Check sheet for the modelled part. Datum: model origin and axes. Units: mm. A direction names the side the tool comes from. Round coordinates to 2 decimals unless told otherwise and drop trailing zeros. Order: outer loops, then holes, each group sorted by start corner. A loop starts at its lowest first (then second) coordinate and runs counter-clockwise, first axis right, second up.
Q1. Cross-section at A-A on y = 0. Record the cut outline in (x, z).
Q2. Set-up check for faces 1 (the flat face through (0, 3, 19)), 2 (the cylindrical face through (-6, 0, 21)), 3 (the flat face through (0, -6, 14)): record each of +Z, -Z, +X, -X, +Y, -Y from which the full face is reachable in a straight line by a thin tool's end or side.
Q3. Scan lines: probe 1 along Y at (x, z) = (13.5, 18.5); probe 2 along Y at (x, z) = (-5, 16); probe 3 along X at (y, z) = (4, 18.75). Record each from-to range of solid material in increasing order.
Q4. Depth check by flat-ended pin: P1, Ø4, axis at x = 0, z = 17.5, coming from the -Y side; P2, Ø2, axis at x = -18, z = 17.5, coming from the +Y side; P3, Ø23, axis at x = -10.58, y = -14.56, coming from the +Z side. Enter the tip coordinate at first touch or a pass-through.
Q5. Cross-section at B-B on x = -13. Give the number of separate pieces and of enclosed holes in the cut face, then the cut area to 3 significant figures.
Q6. Mould release check, pull along Y, two halves, no side actions. Record for faces 4 (the flat face through (-1.42, -3.92, 24)), 5 (the cylindrical face through (-1.302, 27.915, 16.465)), 6 (the cylindrical face through (22.923, -2.581, 16.465)), 7 (the cylindrical face through (-29.97, 1.32, 16.5)): +Y half, -Y half, draft (parallel to the pull), parting line (faces both ways), or undercut.
from build123d import *

# Parameters (mm, degrees)
CYLINDER003_R     = 10
CYLINDER003_DEPTH = 10
ARRAY_COUNT       = 5
TORUS001_R        = 0.8
TORUS_R           = 0.8
CYLINDER_R        = 4
CYLINDER_DEPTH    = 10
BOX_W             = 8
BOX_H             = 7
BOX_DEPTH         = 10
CYLINDER002_R     = 6
CYLINDER002_DEPTH = 10
CYLINDER001_R     = 30
CYLINDER001_DEPTH = 5


with BuildPart() as fusion001:
    # Cylinder003 → Cylinder003 (new body)
    with BuildSketch(Plane(origin=(0, 18, 0), x_dir=(1, 0, 0), z_dir=(0, 0, 1))):
        Circle(CYLINDER003_R)
    extrude(amount=CYLINDER003_DEPTH)

    # Array: Fusion001 ×5 about axis
    array_axis = Axis((0, 0, 0), (0, 0, 1))


with BuildPart() as fusion001_1:
    add(fusion001.part)
    for i in range(1, ARRAY_COUNT):
        add(fusion001.part.rotate(array_axis, i * 360 / ARRAY_COUNT))


with BuildPart() as torus001:
    # Torus001 → Torus001 (revolve)
    with BuildSketch(Plane(origin=(0, 0, 3.5), x_dir=(1, 0, 0), z_dir=(0, -1, 0))):
        with Locations((30, 0)):
            Circle(TORUS001_R)
    revolve(axis=Axis((0, 0, 3.5), (0, 0, 1)))


with BuildPart() as torus:
    # Torus → Torus (revolve)
    with BuildSketch(Plane(origin=(0, 0, 1.5), x_dir=(1, 0, 0), z_dir=(0, -1, 0))):
        with Locations((30, 0)):
            Circle(TORUS_R)
    revolve(axis=Axis((0, 0, 1.5), (0, 0, 1)))


with BuildPart() as cylinder:
    # Cylinder → Cylinder (new body)
    with BuildSketch(Plane.XY):
        Circle(CYLINDER_R)
    extrude(amount=CYLINDER_DEPTH)


with BuildPart() as common:
    # Box → Box (new body)
    with BuildSketch(Plane(origin=(-4, -4, 0), x_dir=(1, 0, 0), z_dir=(0, 0, 1))):
        with Locations((4, 3.5)):
            Rectangle(BOX_W, BOX_H)
    extrude(amount=BOX_DEPTH)

    # Common: intersect Cylinder
    add(cylinder.part, mode=Mode.INTERSECT)


with BuildPart() as cylinder002:
    # Cylinder002 → Cylinder002 (new body)
    with BuildSketch(Plane.XY):
        Circle(CYLINDER002_R)
    extrude(amount=CYLINDER002_DEPTH)


with BuildPart() as cut003:
    # Cylinder001 → Cylinder001 (new body)
    with BuildSketch(Plane.XY):
        Circle(CYLINDER001_R)
    extrude(amount=CYLINDER001_DEPTH)

    # Fusion: union Cylinder002
    add(cylinder002.part)

    # Cut: cut Common
    add(common.part, mode=Mode.SUBTRACT)

    # Cut001: cut Torus
    add(torus.part, mode=Mode.SUBTRACT)

    # Cut002: cut Torus001
    add(torus001.part, mode=Mode.SUBTRACT)

    # Cut003: cut Fusion001
    add(fusion001_1.part, mode=Mode.SUBTRACT)


with BuildPart() as cut003_1:
    # Cut003 placement: moved
    add(cut003.part.moved(Location((0, 0, 14))))


solid = cut003_1.part
Results found:
1. outline: (-30, 14) - (-25.43, 14) - (-25.43, 19) - (-30, 19) - (-30, 18.3) arc R0.8 cw to (-30, 16.7) - (-30, 16.3) arc R0.8 cw to (-30, 14.7) - close; (-8.81, 14) - (-4, 14) - (-4, 24) - (-6, 24) - (-6, 19) - (-8.81, 19) - close; (4, 14) - (8.81, 14) - (8.81, 19) - (6, 19) - (6, 24) - (4, 24) - close; (25.43, 14) - (30, 14) - (30, 14.7) arc R0.8 cw to (30, 16.3) - (30, 16.7) arc R0.8 cw to (30, 18.3) - (30, 19) - (25.43, 19) - close
2. face 1: +Z, -Z
2. face 2: +Z
2. face 3: -Z, +X, -X, +Y, -Y
3. probe 1: y = -26.79 to -24.13, -5 to -3.76, 14.88 to 26.79
3. probe 2: y = -28.95 to -22.86, -6.26 to 9.34, 26.66 to 28.95
3. probe 3: x = -29.73 to -27, -7.24 to 7.24, 27 to 29.73
4. P1: stops at y = -30
4. P2: stops at y = 24.44
4. P3: stops at z = 19
5. separate pieces: 3
5. enclosed holes: 0
5. area: 77.7 mm2
6. face 4: draft
6. face 5: undercut
6. face 6: undercut
6. face 7: parting line
